from build123d import *

# Parameters (mm, degrees)
CROQUIS1_R                    = 17.5
SALIENTE_EXTRUIR1_DEPTH       = 20
TALADRO_ROSCADO_1_4_201_D     = 5.1054
TALADRO_ROSCADO_1_4_201_DEPTH = 19.05
TALADRO_ROSCADO_1_4_201_TIP   = 1.533816902


with BuildPart() as part:
    # Croquis1 → Saliente-Extruir1 (new, symmetric)
    with BuildSketch(Plane.XY):
        Polygon((28, 60), (15, 60), (9.803847577, 63), (-9.803847577, 63), (-15, 60), (-28, 60), (-28, 17), (-30, 15), (-30, 0), (30, 0), (30, 15), (28, 17), align=None)
        with Locations((0, 30)):
            Circle(CROQUIS1_R, mode=Mode.SUBTRACT)
    extrude(amount=SALIENTE_EXTRUIR1_DEPTH, both=True)

    # Taladro roscado 1/4-201
    with Locations(Plane(origin=(0, 0, 0), x_dir=(-1, 0, 0), z_dir=(0, -1, 0))):
        with Locations((20, 10), (20, -10), (-20, -10), (-20, 10)):
            Hole(TALADRO_ROSCADO_1_4_201_D / 2, depth=TALADRO_ROSCADO_1_4_201_DEPTH)
            with Locations((0, 0, -(TALADRO_ROSCADO_1_4_201_DEPTH + TALADRO_ROSCADO_1_4_201_TIP / 2))):  # 118° drill point
                Cone(0, TALADRO_ROSCADO_1_4_201_D / 2, TALADRO_ROSCADO_1_4_201_TIP, mode=Mode.SUBTRACT)


solid = part.part
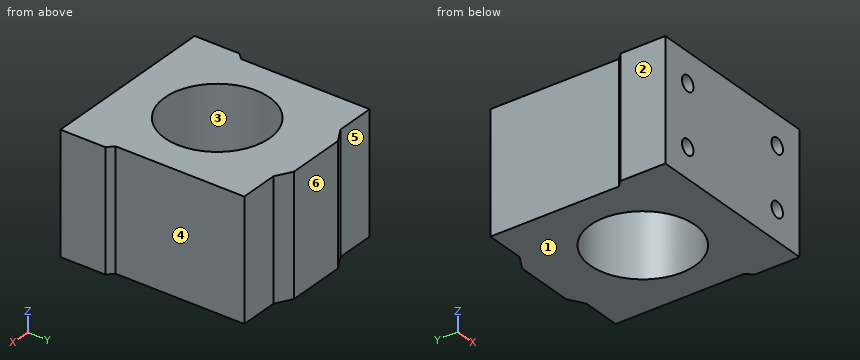
Verification items for the finished model (mm, model axes). Face numbers are marked on the shaded views. A direction names the side the tool comes from. Round coordinates to 2 decimals unless told otherwise and drop trailing zeros. Loops run counter-clockwise (first coordinate to the right, second up) from the corner with the lowest first, then second, coordinate; pieces in that order, holes last. Notation, with made-up numbers: (-14, 83.25) - (29, 83.25) arc R26 cw to (29, 109.25) - close; hole circle Ø9 at (-17.5, -21.75). An arc over 180 degrees is marked (long way). Use a Markdown table: item, result. Add a question column.
1. Section check D-D, the plane y = 7.5. Record the boundary of the cut face in (x, z), plus the area to 3 significant figures.
2. Section check A-A, the plane y = 30. Record the boundary of the cut face in (x, z).
3. Section check C-C, the plane z = -4. Record the boundary of the cut face in (x, y).
4. Section check B-B, the plane x = 0. Record the boundary of the cut face in (y, z), plus the area to 3 significant figures.
5. Release check for a two-part mould opening along X. For the marked faces 1, 2 and 3 record: released by +X, released by -X, zero draft, split by the parting line, or undercut.
6. Access from +Z, -Z, +X, -X, +Y, -Y to the whole of each face (thin tool, end or side, straight path). Record for the marked faces 4, 5 and 6.
7. Thickness scan on probe 1 along X at (y, z) = (11.25, -10); probe 2 along Z at (x, y) = (-20, 6.5); probe 3 along X at (y, z) = (21, 13.5). Record the ranges inside material, lowest first. Write a range as [from, to].
8. Gauge pin test, flat ends, axial feed: pin 1 (6.5 mm diameter, centred on x = -20, z = -10, fed in from +Y); pin 2 (3 mm diameter, centred on x = 12.5, z = 0.5, fed in from +Y); pin 3 (12 mm diameter, centred on y = 38, z = -8, fed in from -X). Record the tip position at first contact, or that the pin passes through.
Checks:
| question | item | result |
|---|---|---|
| 1 | outline | (-30, -20) - (30, -20) - (30, 20) - (-30, 20) - close; hole circle Ø5.11 at (-20, -10); hole circle Ø5.11 at (-20, 10); hole circle Ø5.11 at (20, -10); hole circle Ø5.11 at (20, 10) |
| 1 | area | 2,320 mm^2 |
| 2 | outline | (-28, -20) - (-17.5, -20) - (-17.5, 20) - (-28, 20) - close; (17.5, -20) - (28, -20) - (28, 20) - (17.5, 20) - close |
| 3 | outline | (-30, 0) - (30, 0) - (30, 15) - (28, 17) - (28, 60) - (15, 60) - (9.8, 63) - (-9.8, 63) - (-15, 60) - (-28, 60) - (-28, 17) - (-30, 15) - close; hole circle Ø35 at (0, 30) |
| 4 | outline | (0, -20) - (12.5, -20) - (12.5, 20) - (0, 20) - close; (47.5, -20) - (63, -20) - (63, 20) - (47.5, 20) - close |
| 4 | area | 1,120 mm^2 |
| 5 | face 1 | zero draft |
| 5 | face 2 | released by -X |
| 5 | face 3 | undercut |
| 6 | face 4 | +Z, -Z, +X, +Y |
| 6 | face 5 | +Z, -Z, -X, +Y |
| 6 | face 6 | +Z, -Z, +X, -X, +Y |
| 7 | probe 1 | x = [-30, -22.55], [-17.45, 17.45], [22.55, 30] |
| 7 | probe 2 | z = [-20, -12.55], [-7.45, 7.45], [12.55, 20] |
| 7 | probe 3 | x = [-28, -15.01], [15.01, 28] |
| 8 | pin 1 | stops at y = 60 |
| 8 | pin 2 | stops at y = 62.31 |
| 8 | pin 3 | stops at x = -28 |
